from build123d import *

# Parameters (mm, degrees)
SKETCH1_R           = 1.5
BOSS_EXTRUDE1_DEPTH = 4
CUT_EXTRUDE2_DEPTH  = 5
CIRPATTERN1_COUNT   = 12
SKETCH3_W           = 7.863082298
SKETCH3_H           = 5
BOSS_EXTRUDE2_DEPTH = 4
SKETCH4_R           = 2.5
CUT_EXTRUDE3_DEPTH  = 5


with BuildPart() as part:
    # Sketch1 → Boss-Extrude1 (new body)
    with BuildSketch(Plane.XY):
        with BuildLine():
            Line((-18, 2.5), (12.545643943, 2.5))
            ThreePointArc((12.545643943, 2.5), (24, 0), (12.545643943, -2.5))
            Line((12.545643943, -2.5), (-18, -2.5))
            ThreePointArc((-18, -2.5), (-20.5, 0), (-18, 2.5))
        make_face()
        with Locations((-18, 0)):
            Circle(SKETCH1_R, mode=Mode.SUBTRACT)
    extrude(amount=BOSS_EXTRUDE1_DEPTH)

    # Sketch2 → Cut-Extrude2 (cut, through all)
    with BuildSketch(Plane.XY.offset(4)):
        with BuildLine():
            Line((18.72, 5.06), (18.653012702, 4.81))
            ThreePointArc((18.653012702, 4.81), (19.09327028, 4.061267387), (19.842002893, 4.501524965))
            Line((19.842002893, 4.501524965), (19.906461709, 4.742088543))
            ThreePointArc((19.906461709, 4.742088543), (20.342188248, 5.236548367), (21, 5.196152423))
            ThreePointArc((21, 5.196152423), (19.615923505, 6.030708621), (18, 6))
            ThreePointArc((18, 6), (18.589879661, 5.706078038), (18.72, 5.06))
        make_face()
    cut_extrude2 = extrude(amount=-CUT_EXTRUDE2_DEPTH, mode=Mode.SUBTRACT)

    # CirPattern1: Cut-Extrude2 ×12 about axis
    cirpattern1_axis = Axis((18, 0, 0), (0, 0, 1))
    for i in range(1, CIRPATTERN1_COUNT):
        add(cut_extrude2.rotate(cirpattern1_axis, i * 360 / CIRPATTERN1_COUNT), mode=Mode.SUBTRACT)

    # Sketch3 → Boss-Extrude2 (add)
    with BuildSketch(Plane.XY.offset(4)):
        with Locations((12.029323846, 0)):
            Rectangle(SKETCH3_W, SKETCH3_H)
    extrude(amount=-BOSS_EXTRUDE2_DEPTH)

    # Sketch4 → Cut-Extrude3 (cut, through all)
    with BuildSketch(Plane.XY.offset(4)):
        with Locations((18, 0)):
            Circle(SKETCH4_R)
    extrude(amount=-CUT_EXTRUDE3_DEPTH, mode=Mode.SUBTRACT)


solid = part.part
Can you work these out from the model? Positions are in its coordinate system, mm. Give positions to 0.01 mm unless a question says otherwise; leave off trailing zeros. Return JSON: item names as keys, results as strings.
Q1. We'd pull the mould along X, two halves only. Please class faces 1 (the face through (15.02, 2.97, 2.03)), 2 (the face through (21.363, 4.656, 2.028)), 3 (the face through (4, 0, 4)), 4 (the face through (14.637, -4.656, 2.028)): released by +X, released by -X, zero draft, split by the parting line, or undercut.
Checks:
{"face 1": "undercut", "face 2": "released by +X", "face 3": "zero draft", "face 4": "released by -X"}
Q2. I need wall thicknesses on probe 1 along Y at (x, z) = (18, 1.3); probe 2 along X at (y, z) = (-0.25, 1.5); probe 3 along X at (y, z) = (-1, 2.3). Which ranges of each line are inside material? Lowest first, please.
Checks:
{"probe 1": "y = -6 to -2.5, 2.5 to 6", "probe 2": "x = -20.49 to -19.48, -16.52 to 15.51, 20.49 to 23.96", "probe 3": "x = -20.29 to -19.12, -16.88 to 15.71, 20.29 to 22.09"}
Q3. For pin 1 Ø1 at (x, z) = (-7.5, 0.5) entering from +Y; pin 2 Ø1.2 at (x, z) = (-9.5, 2.5) entering from -Y, each with a flat end and sliding along its axis, tell me the tip position at first contact or that it passes through.
Checks:
{"pin 1": "stops at y = 2.5", "pin 2": "stops at y = -2.5"}
Q4. I want a section at A-A, the plane z = 1.65. Count the separate pieces of the cut face and the enclosed holes in it, then the cut area to 3 significant figures.
Checks:
{"separate pieces": "1", "enclosed holes": "2", "area": "223 mm2"}
